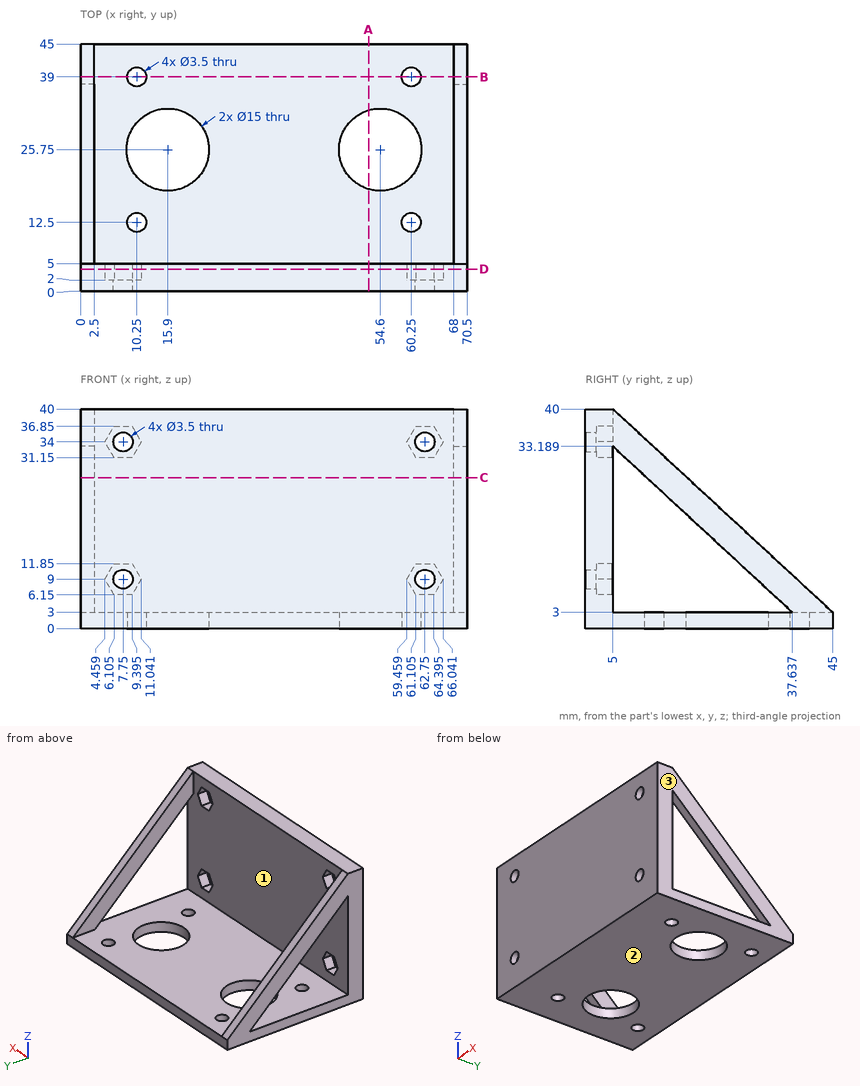
Answer from the drawing. Dimensions are ordinates in mm from the lowest x, y and z of the part. Coordinates: 2 decimals unless noted, no trailing zeros. Write each loop counter-clockwise with the first axis right and the second up, starting at its lowest first coordinate (ties: lowest second). Pieces come first, ordered by that corner, then holes. Notation, with made-up numbers: M -3.75,20 L 17.25,20 A19 ccw 17.25,50 Z; hole C 36,79.5 d6. An arc over 180 degrees is marked long. Use one line per item in the form item = value. Start each with the question number.
1. The part is cut by section B-B (y = 39). Give the vertices of the cut face in (x, z), plus the area to 3 significant figures.
2. Straight lines are drawn through the part: probe 1 along X at (y, z) = (1, 9); probe 2 along Z at (x, y) = (7.75, 0.85); probe 3 along Z at (x, y) = (62, 1). For each, find the intervals that lie inside material, in ascending order. Write a range as from..to.
3. Each of these flat-tipped pins is pushed along its axis until it touches: P1, Ø3, axis at x = 60.25, y = 39, coming from the -Z side; P2, Ø8, axis at x = 25.5, z = 21.5, coming from the +Y side; P3, Ø4.5, axis at x = 62.5, z = 34.5, coming from the +Y side. Where does it stop, or does it pass through?
4. The mould has two halves that part along X. Classify the marked faces 1, 2 and 3: released by +X, released by -X, zero draft, split by the parting line, or undercut.
5. The part is cut by section A-A (x = 52.5). Give the vertices of the cut face in (y, z), plus the area to 3 significant figures.
6. The part is cut by section D-D (y = 4). Give the number of separate pieces and of enclosed holes in the cut face, plus the area to 3 significant figures.
7. The part is cut by section C-C (z = 27.5). Give the vertices of the cut face in (x, y), plus the area to 3 significant figures.
Evaluation:
q1.outline = M 0,0 L 8.5,0 L 8.5,3 L 2.5,3 L 2.5,8.55 L 0,8.55 Z; M 12,0 L 58.5,0 L 58.5,3 L 12,3 Z; M 62,0 L 70.5,0 L 70.5,8.55 L 68,8.55 L 68,3 L 62,3 Z
q1.area = 218 mm^2
q2.probe_1 = 0..6, 9.5..61, 64.5..70.5
q2.probe_2 = 0..7.25, 10.75..32.25, 35.75..40
q2.probe_3 = 0..7.42, 10.58..32.42, 35.58..40
q3.P1 = through
q3.P2 = 5
q3.P3 = 2
q4.face_1 = undercut
q4.face_2 = zero draft
q4.face_3 = released by +X
q5.outline = M 0,0 L 18.55,0 L 18.55,3 L 5,3 L 5,40 L 0,40 Z; M 32.95,0 L 45,0 L 45,3 L 32.95,3 Z
q5.area = 277 mm^2
q6.separate_pieces = 1
q6.enclosed_holes = 4
q6.area = 2,710 mm^2
q7.outline = M 0,0 L 70.5,0 L 70.5,5 L 0,5 Z; M 0,11.15 L 2.5,11.15 L 2.5,18.51 L 0,18.51 Z; M 68,11.15 L 70.5,11.15 L 70.5,18.51 L 68,18.51 Z
q7.area = 389 mm^2
